For this review, take the finished solid that the model builds, in its own axes (mm). A direction names the side the tool comes from. Give positions to 0.01 mm unless a question says otherwise; leave off trailing zeros. Write each loop counter-clockwise with the first axis right and the second up, starting at its lowest first coordinate (ties: lowest second). Pieces come first, ordered by that corner, then holes.
1) Draft analysis for pull direction Y (two halves, no side actions). For faces 4 (the face through (-8.5, 0, 6)), 5 (the face through (-13.944, -25.505, 0.813)), 6 (the face through (0, 8.5, 6)), state which applies: pulls with the +Y half, pulls with the -Y half, needs draft (parallel to the pull), parting line crosses it, or undercut.
2) We need section B-B on y = -26.08. Give the boundary of the cut face in (x, z), and give its area (3 significant figures).
3) For P1, Ø4, axis at x = -15.33, y = -26.08, coming from the +Z side; P2, Ø4, axis at x = 15.33, y = 6.92, coming from the -Z side; P3, Ø4, axis at y = -5.5, z = 22.5, coming from the +X side; P4, Ø4, axis at y = -3.5, z = 6, coming from the -X side, all flat-tipped, find the tip position at first contact; note any pin that passes through.
4) We need section D-D on y = 6.92. Give the boundary of the cut face in (x, z).
5) We need section A-A on x = -15.33. Give the boundary of the cut face in (y, z).
6) Machinability: for faces 1 (the face through (-8, 0, 9.65)), 2 (the face through (8.5, 0, 6)), 3 (the face through (0, -8.5, 6)), which of the approach directions +Z, -Z, +X, -X, +Y, -Y give a long, thin tool a straight path to every point of the face, cutting with its end or side? Answer none if there is none.
7) We need section C-C on x = 15.33. Give the boundary of the cut face in (y, z), and give its area (3 significant figures).
8) Wall thickness on line 1 along Y through (x, z) = (-15.33, 0.75); line 2 along Y through (x, z) = (15.33, 1.15); line 3 along Z through (x, y) = (10.5, -4.5): over which ranges is each line inside the solid? List them lowest first.
Autodesk Inventor part; units mm, degrees
ref_plane "YZ Plane" through (0, 0, 0) normal (1, 0, 0) x (0, 1, 0)
ref_plane "XZ Plane" through (0, 0, 0) normal (0, 1, 0) x (-1, 0, 0)
ref_plane "XY Plane" through (0, 0, 0) normal (0, 0, 1) x (1, 0, 0)
sketch "Sketch1" plane through (0, 0, 0) normal (0, 0, 1) x (1, 0, 0)
  line L0 (0, 0) -> (0, 8.5)
  line L1 (0, 8.5) -> (8.5, 8.5)
  line L2 (8.5, 8.5) -> (8.5, -8.5)
  line L3 (8.5, -8.5) -> (-8.5, -8.5)
  line L4 (-8.5, -8.5) -> (-8.5, 8.5)
  line L5 (-8.5, 8.5) -> (0, 8.5)
  line L6 (0, 8.5) -> (0, 10.25)
  line L7 (0, 10.25) -> (-15.33, 10.25)
  line L8 (-15.33, 10.25) -> (-15.33, 6.92)
  circle A0 centre (-15.33, 6.92) radius 1.5
  line L9 (0, 10.25) -> (15.33, 10.25)
  line L10 (15.33, 10.25) -> (15.33, 6.92)
  circle A1 centre (15.33, 6.92) radius 1.5
  line L11 (-15.33, 6.92) -> (-15.33, -26.08)
  circle A2 centre (-15.33, -26.08) radius 1.5
  line L12 (0, 0) -> (0, 6.92)
  line L13 (-16.83, 6.92) -> (-18.08, 6.92)
  line L14 (-18.08, 6.92) -> (-18.08, -28.83)
  line L15 (-18.08, 6.92) -> (-18.08, 11.5)
  line L16 (-18.08, 11.5) -> (-3.5327, 11.5)
  line L17 (-3.5327, 11.5) -> (18.0803, 11.5)
  line L18 (18.0803, 11.5) -> (18.0803, -28.83)
  line L19 (18.0803, -28.83) -> (-18.08, -28.83)
  dimension "d8" = 3
  dimension "d0" = 8.5
  dimension "d1" = 8.5
  dimension "d2" = 17
  dimension "d3" = 17
  dimension "d4" = 17
  dimension "d5" = 1.75
  dimension "d6" = 15.33
  dimension "d7" = 3.33
  dimension "d9" = 15.33
  dimension "d10" = 3.33
  dimension "d11" = 3
  dimension "d12" = 33
  dimension "d13" = 3
  dimension "d14" = 1.25
  dimension "d15" = 35.75
  dimension "d16" = 4.58
  dimension "d17" = 21.613
extrude "Extrusion1" add sketch "Sketch1" along normal blind 1.65
sketch "Sketch2" plane through (0, 0, 1.65) normal (0, 0, 1) x (1, 0, 0)
  line L0 (-8.5, 8.5) -> (-8.5, -8.5)
  line L1 (8.5, 8.5) -> (8.5, -8.5)
  line L2 (-8.5, 8.5) -> (8.5, 8.5)
  line L3 (8.5, 8.5) -> (8.5, -8.5)
  line L4 (8.5, -8.5) -> (-8.5, -8.5)
  line L5 (-8.5, -8.5) -> (-8.5, 8.5)
  point P0 (0, 0)
extrude "Extrusion2" add sketch "Sketch2" along normal blind 8 and the other way blind 1.65
sketch "Sketch3" plane through (0, 0, 9.65) normal (0, 0, 1) x (1, 0, 0)
  circle A0 centre (0, 0) radius 7.5
  dimension "d24" = 15
extrude "Extrusion3" add sketch "Sketch3" along normal blind 16
properties part number "Pixy Sketch"
Results list:
1. face 4: needs draft
1. face 5: undercut
1. face 6: pulls with the +Y half
2. outline: (-18.08, 0) - (-16.83, 0) - (-16.83, 1.65) - (-18.08, 1.65) - close; (-13.83, 0) - (18.08, 0) - (18.08, 1.65) - (-13.83, 1.65) - close
2. area: 54.7 mm2
3. P1: stops at z = 1.65
3. P2: stops at z = 0
3. P3: stops at x = 6.63
3. P4: stops at x = -8.5
4. outline: (-18.08, 0) - (-16.83, 0) - (-16.83, 1.65) - (-18.08, 1.65) - close; (-13.83, 0) - (13.83, 0) - (13.83, 1.65) - (8.5, 1.65) - (8.5, 9.65) - (2.89, 9.65) - (2.89, 25.65) - (-2.89, 25.65) - (-2.89, 9.65) - (-8.5, 9.65) - (-8.5, 1.65) - (-13.83, 1.65) - close; (16.83, 0) - (18.08, 0) - (18.08, 1.65) - (16.83, 1.65) - close
5. outline: (-28.83, 0) - (-27.58, 0) - (-27.58, 1.65) - (-28.83, 1.65) - close; (-24.58, 0) - (5.42, 0) - (5.42, 1.65) - (-24.58, 1.65) - close; (8.42, 0) - (11.5, 0) - (11.5, 1.65) - (8.42, 1.65) - close
6. face 1: +Z
6. face 2: +Z, +X, +Y, -Y
6. face 3: +Z, +X, -X, -Y
7. outline: (-28.83, 0) - (5.42, 0) - (5.42, 1.65) - (-28.83, 1.65) - close; (8.42, 0) - (11.5, 0) - (11.5, 1.65) - (8.42, 1.65) - close
7. area: 61.6 mm2
8. line 1: y = -28.83 to -27.58, -24.58 to 5.42, 8.42 to 11.5
8. line 2: y = -28.83 to 5.42, 8.42 to 11.5
8. line 3: z = 0 to 1.65
